The figure shows three views and two pictorial views of one solid part (mm, origin at its lowest corner). Answer the questions. A direction names the side the tool comes from. Coordinates: 2 decimals unless noted, no trailing zeros. Order: outer loops, then holes, each group sorted by start corner. A loop starts at its lowest first (then second) coordinate and runs counter-clockwise, first axis right, second up. Notation, with made-up numbers: (61, 77) - (78, 77) arc R20 cw to (78, 84) - close; hole circle Ø1 at (-14.75, -25.75). An arc over 180 degrees is marked (long way). Use one line per item in the form item = value. Start each with the question number.
Item 1: Consider line 1 along Y through (x, z) = (25, 18); line 2 along Z through (x, y) = (9, 11.5); line 3 along Y through (x, z) = (8.5, 26). Determine where each line is inside the solid, lowest interval first. Write a range as [from, to].
Item 2: Section D-D, the plane x = 49.5 is taken. Write down the section's boundary in (y, z), and give its area (3 significant figures).
Item 3: Section A-A, the plane x = 18 is taken. Write down the section's boundary in (y, z) (1 decimal), and give its area (3 significant figures).
Item 4: The mould has two halves that part along Y. Classify the marked faces 4, 5 and 6: released by +Y, released by -Y, zero draft, split by the parting line, or undercut.
Item 5: Each of these flat-tipped pins is pushed along its axis until it touches: pin 1 Ø1.5 at (x, y) = (44.5, 37) entering from -Z; pin 2 Ø25 at (x, y) = (33, 37) entering from +Z; pin 3 Ø10.5 at (x, z) = (41, 40) entering from -Y. Where does it stop, or does it pass through?
Item 6: Section B-B, the plane y = 31.5 is taken. Write down the section's boundary in (x, z) (1 decimal).
Item 7: A tool of negligible diameter and unlimited length cuts with its end or side. For the marked faces 1, 2 and 3, from which of +Z, -Z, +X, -X, +Y, -Y can it reach the whole face along a straight path? Write none if from no direction.
Item 8: Section C-C, the plane z = 36 is taken. Write down the section's boundary in (x, y) (1 decimal), and give its area (3 significant figures).
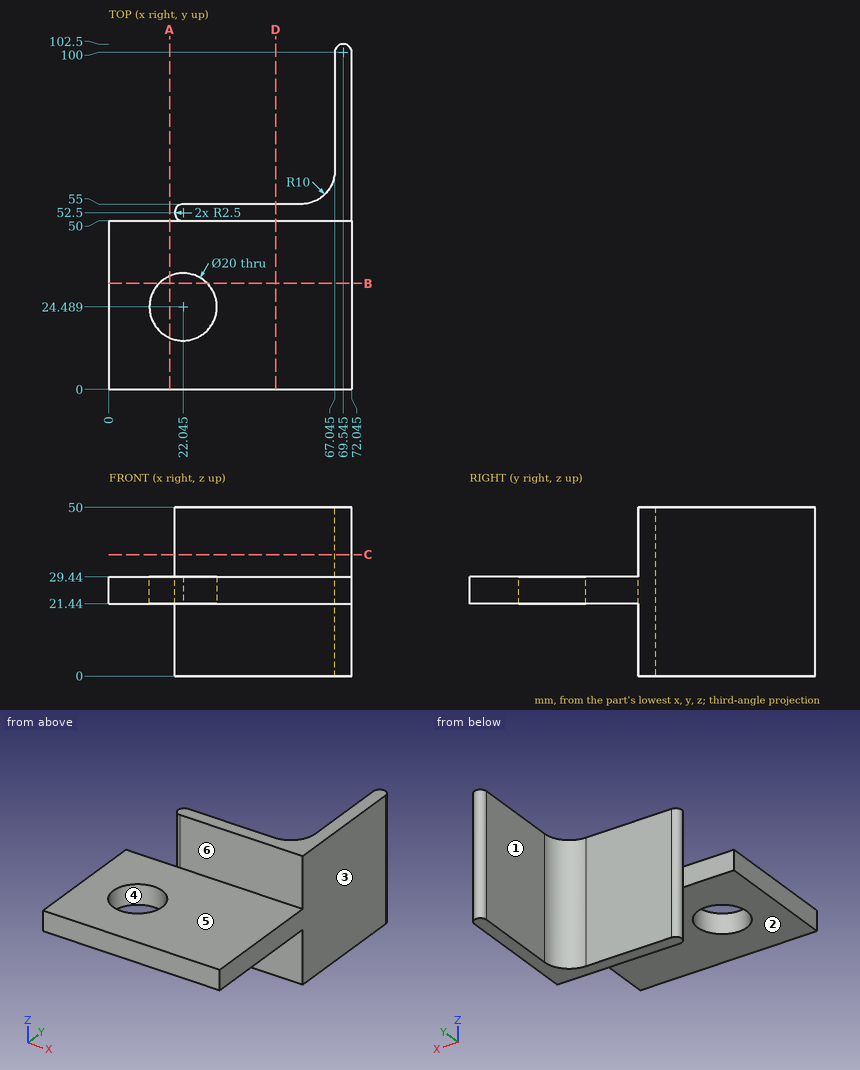
Response:
q1.line_1 = [50, 55]
q1.line_2 = [21.44, 29.44]
q1.line_3 = [0, 50]
q2.outline = (0, 21.44) - (50, 21.44) - (50, 0) - (55, 0) - (55, 50) - (50, 50) - (50, 29.44) - (0, 29.44) - close
q2.area = 650 mm2
q3.outline = (0, 21.4) - (15.3, 21.4) - (15.3, 29.4) - (0, 29.4) - close; (33.6, 21.4) - (50, 21.4) - (50, 29.4) - (33.6, 29.4) - close
q3.area = 254 mm2
q4.face_4 = undercut
q4.face_5 = zero draft
q4.face_6 = released by -Y
q5.pin_1 = 21.44
q5.pin_2 = 29.44
q5.pin_3 = 50
q6.outline = (0, 21.4) - (14.9, 21.4) - (14.9, 29.4) - (0, 29.4) - close; (29.2, 21.4) - (72, 21.4) - (72, 29.4) - (29.2, 29.4) - close
q7.face_1 = +Z, -Z, -X, +Y
q7.face_2 = -Z, +X, -X, -Y
q7.face_3 = +Z, -Z, +X, +Y, -Y
q8.outline = (22, 50) - (72, 50) - (72, 100) arc R2.5 ccw to (67, 100) - (67, 65) arc R10 cw to (57, 55) - (22, 55) arc R2.5 ccw to start
q8.area = 516 mm2
